```python
from build123d import *

# Parameters (mm, degrees)
BOSS_EXTRUDE1_DEPTH    = 15
SKETCH1_5_W            = 7.4
SKETCH1_5_H            = 7.4
BOSS_EXTRUDE2_DEPTH    = 7
CHAMFER1_SIZE          = 1
SKETCH2_R              = 9.708243919
SKETCH2_R_2            = 4
INNER_DISK_DEPTH       = 5
HOLE_DEPTH             = 65.033705881
HOLE_DEPTH_BACK        = 65.033705881
CUT_EXTRUDE5_DEPTH     = 6
CUT_EXTRUDE3_DEPTH     = 4
CUT_EXTRUDE4_START     = -8.25
CUT_EXTRUDE4_OUTLINE_W = 25.326781011
CUT_EXTRUDE4_OUTLINE_H = 3
CUT_EXTRUDE4_DEPTH     = 3


# Read off the part's stored shape, not the designer's step: Cut-Extrude4
with BuildPart() as part:
    # Sketch1 → Boss-Extrude1 (new body)
    with BuildSketch(Plane.XY):
        Polygon((30, 0), (13.753072731, 52.118283633), (-13.753072731, 52.118283633), (-30, 0), (-15, -48.118283633), (15, -48.118283633), align=None)
    extrude(amount=BOSS_EXTRUDE1_DEPTH)

    # Sketch1<5> → Boss-Extrude2 (add)
    with BuildSketch(Plane.XY):
        with Locations((10.003072731, 33.468283633)):
            Rectangle(SKETCH1_5_W, SKETCH1_5_H)
        with Locations((-11.25, -29.468283633)):
            Rectangle(SKETCH1_5_W, SKETCH1_5_H)
    extrude(amount=-BOSS_EXTRUDE2_DEPTH)

    # Chamfer1
    chamfer1_edges = [part.edges().sort_by_distance(p)[0] for p in [
        (10.003072731, 37.168283633, -7),
        (6.303072731, 33.468283633, -7),
        (13.703072731, 33.468283633, -7),
        (10.003072731, 29.768283633, -7),
        (-11.25, -33.168283633, -7),
        (-7.55, -29.468283633, -7),
        (-14.95, -29.468283633, -7),
        (-11.25, -25.768283633, -7),
    ]]
    chamfer(chamfer1_edges, length=CHAMFER1_SIZE)

    # Sketch2 → Inner Disk (cut)
    with BuildSketch(Plane(origin=(0, 0, 0), x_dir=(-1, 0, 0), z_dir=(0, 0, -1))):
        Circle(SKETCH2_R)
        Circle(SKETCH2_R_2, mode=Mode.SUBTRACT)
    extrude(amount=-INNER_DISK_DEPTH, mode=Mode.SUBTRACT)

    # Sketch3 → Hole (cut, two sides: drawn at the far end of the back side and taken through both)
    with BuildSketch(Plane.XY.offset(15).offset(-HOLE_DEPTH_BACK)):
        with BuildLine():
            ThreePointArc((-15, 23), (-20.5, 17.5), (-15, 12))
            Line((-15, 12), (-15, 17.5))
            Line((-15, 17.5), (-15, 23))
        make_face()
        with BuildLine():
            Line((-15, 17.5), (-15, 12))
            ThreePointArc((-15, 12), (-11.110912703, 13.610912703), (-9.5, 17.5))
            ThreePointArc((-9.5, 17.5), (-11.110912703, 21.389087297), (-15, 23))
            Line((-15, 23), (-15, 17.5))
        make_face()
        with BuildLine():
            ThreePointArc((-9.5, -17.5), (-11.110912703, -13.610912703), (-15, -12))
            Line((-15, -12), (-15, -17.5))
            Line((-15, -17.5), (-15, -23))
            ThreePointArc((-15, -23), (-11.110912703, -21.389087297), (-9.5, -17.5))
        make_face()
        with BuildLine():
            Line((-15, -17.5), (-15, -12))
            ThreePointArc((-15, -12), (-20.5, -17.5), (-15, -23))
            Line((-15, -23), (-15, -17.5))
        make_face()
    extrude(amount=HOLE_DEPTH + HOLE_DEPTH_BACK, mode=Mode.SUBTRACT)

    # Sketch3<3> → Cut-Extrude5 (cut)
    with BuildSketch(Plane.XY.offset(15)):
        with BuildLine():
            ThreePointArc((-27.063244683, 9.420775021), (-21.167946858, 11.347988345), (-15, 12))
            ThreePointArc((-15, 12), (-20.5, 17.5), (-15, 23))
            Line((-15, 23), (-22.830168203, 23))
            Line((-22.830168203, 23), (-27.063244683, 9.420775021))
        make_face()
    extrude(amount=-CUT_EXTRUDE5_DEPTH, mode=Mode.SUBTRACT)

    # Sketch4 → Cut-Extrude3 (cut)
    with BuildSketch(Plane(origin=(0, 0, 0), x_dir=(-1, 0, 0), z_dir=(0, 0, -1))):
        with BuildLine():
            Line((0, 9.708243919), (0, -2))
            Line((0, -2), (9.5, -2))
            ThreePointArc((9.5, -2), (9.656042596, -1.005406078), (9.708243919, 0))
            ThreePointArc((9.708243919, 0), (6.864765109, 6.864765109), (0, 9.708243919))
        make_face()
        with BuildLine():
            ThreePointArc((9.708243919, 0), (9.656042596, -1.005406078), (9.5, -2))
            Line((9.5, -2), (13.5, -2))
            Line((13.5, -2), (13.5, 12.208497378))
            ThreePointArc((13.5, 12.208497378), (9.5, 17.5), (13.5, 22.791502622))
            Line((13.5, 22.791502622), (13.5, 26.791502622))
            Line((13.5, 26.791502622), (8.25, 26.791502622))
            Line((8.25, 26.791502622), (5.25, 26.791502622))
            Line((5.25, 26.791502622), (0, 26.791502622))
            Line((0, 26.791502622), (0, 17.5))
            Line((0, 17.5), (0, 9.708243919))
            ThreePointArc((0, 9.708243919), (6.864765109, 6.864765109), (9.708243919, 0))
        make_face()
    extrude(amount=-CUT_EXTRUDE3_DEPTH, mode=Mode.SUBTRACT)

    # Cut-Extrude4 outline → Cut-Extrude4 (cut)
    with BuildSketch(Plane.YZ.offset(CUT_EXTRUDE4_START)):
        with Locations((39.454893128, 1.5)):
            Rectangle(CUT_EXTRUDE4_OUTLINE_W, CUT_EXTRUDE4_OUTLINE_H)
    extrude(amount=CUT_EXTRUDE4_DEPTH, mode=Mode.SUBTRACT)


solid = part.part
```
The listing builds one solid part. Answer for the finished solid, in the listing's coordinates (mm). A direction names the side the tool comes from. Give positions to 0.01 mm unless a question says otherwise; leave off trailing zeros. Write each loop counter-clockwise with the first axis right and the second up, starting at its lowest first coordinate (ties: lowest second). Pieces come first, ordered by that corner, then holes. Notation, with made-up numbers: M -35,55 L -13,55 A23 cw -13,93 Z; hole C 76.25,-14.5 d3. An arc over 180 degrees is marked long. Write each question's results on one line, items separated by ' | '.
Q1. Section B-B, the plane y = -14 is taken. Write down the section's boundary in (x, z).
Output values:
outline: M -25.64,0 L -19.24,0 L -19.24,15 L -25.64,15 Z; M -10.76,0 L 25.64,0 L 25.64,15 L -10.76,15 Z
Q2. Consider L1, parallel to X at y = 0, z = 2.2; L2, parallel to Z at x = -10, y = 8; L3, parallel to Z at x = -7, y = 37. Determine where each line is inside the solid, lowest interval first. Write a range as from..to.
Output values:
L1: -30..-13.5, 0..4, 9.71..30 | L2: 4..15 | L3: 3..15
Q3. Section A-A, the plane x = -18.5 is taken. Write down the section's boundary in (y, z).
Output values:
outline: M -36.89,0 L -21.74,0 L -21.74,15 L -36.89,15 Z; M -13.26,0 L 13.26,0 L 13.26,9 L 11.79,9 L 11.79,15 L -13.26,15 Z; M 21.74,0 L 36.89,0 L 36.89,15 L 23,15 L 23,9 L 21.74,9 Z
Q4. A tool of negligible diameter and unlimited length cuts with its end or side. For faces 1 (the flat face through (-22, 16, 9)), 2 (the flat face through (-11, -2, 2)), 3 (the flat face through (-8.25, 39, 2)), from which of +Z, -Z, +X, -X, +Y, -Y can it reach the whole face along a straight path? Write none if from no direction.
Output values:
face 1: +Z, -X | face 2: -Z | face 3: -Z, +Y
Q5. Flat-ended cylindrical pins translate along their axes: P1, Ø1.8, axis at y = 32.5, z = -1.5, coming from the -X side; P2, Ø2, axis at y = 19, z = 2.5, coming from the -X side; P3, Ø5, axis at y = -31, z = -3.5, coming from the +X side. Find the tip coordinate at first contact, or state that the pin passes through.
Output values:
P1: x = 6.3 | P2: x = -24.39 | P3: x = -7.55
Q6. Section C-C, the plane x = 5 is taken. Write down the section's boundary in (y, z), then the cut area to 3 significant figures.
Output values:
outline: M -48.12,0 L -8.32,0 L -8.32,5 L 8.32,5 L 8.32,0 L 52.12,0 L 52.12,15 L -48.12,15 Z | area: 1,420 mm2
Q7. For a pull along X with two mould halves and no side action, classify faces 4 (the flat face through (-11, -33.168, -3)), 5 (the cylindrical face through (3.2, -2.4, 2.5)), 6 (the flat face through (6.303, 33, -3)) as released by +X, released by -X, zero draft, split by the parting line, or undercut.
Output values:
face 4: zero draft | face 5: undercut | face 6: released by -X
Q8. Section D-D, the plane y = -29.5 is taken. Write down the section's boundary in (x, z).
Output values:
outline: M -20.8,0 L -14.95,0 L -14.95,-6 L -13.95,-7 L -8.55,-7 L -7.55,-6 L -7.55,0 L 20.8,0 L 20.8,15 L -20.8,15 Z
